```python
from build123d import *

# Parameters (mm, degrees)
SKETCH1_W           = 63.5
SKETCH1_H           = 38.1
BOSS_EXTRUDE1_DEPTH = 8.89
SKETCH2_R           = 2.4638
SKETCH2_R_2         = 1.5875
CUT_EXTRUDE1_DEPTH  = 7.366
SKETCH3_R           = 2.4638
SKETCH3_R_2         = 1.5875
CUT_EXTRUDE2_DEPTH  = 75.584798049


with BuildPart() as part:
    # Sketch1 → Boss-Extrude1 (new body)
    with BuildSketch(Plane(origin=(0, 0, 0), x_dir=(1, 0, 0), z_dir=(0, 1, 0))):
        with Locations((31.75, 19.05)):
            Rectangle(SKETCH1_W, SKETCH1_H)
    extrude(amount=BOSS_EXTRUDE1_DEPTH)

    # Sketch2 → Cut-Extrude1 (cut)
    # profile 1 of 6: a face of its own
    with BuildSketch(Plane(origin=(0, 8.89, 0), x_dir=(1, 0, 0), z_dir=(0, 1, 0))):
        Polygon((17.576011698, 25.4), (15.138005849, 29.62275), (10.261994151, 29.62275), (7.823988302, 25.4), (10.261994151, 21.17725), (15.138005849, 21.17725), align=None)
        with Locations(Location((12.7, 25.4, 0), (0, 0, 270))):
            Circle(SKETCH2_R, mode=Mode.SUBTRACT)
    # profile 2 of 6: a face of its own
    with BuildSketch(Plane(origin=(0, 8.89, 0), x_dir=(1, 0, 0), z_dir=(0, 1, 0))):
        Polygon((36.626011698, 25.4), (34.188005849, 29.62275), (29.311994151, 29.62275), (26.873988302, 25.4), (29.311994151, 21.17725), (34.188005849, 21.17725), align=None)
        with Locations(Location((31.75, 25.4, 0), (0, 0, 270))):
            Circle(SKETCH2_R, mode=Mode.SUBTRACT)
    # profile 3 of 6: a face of its own
    with BuildSketch(Plane(origin=(0, 8.89, 0), x_dir=(1, 0, 0), z_dir=(0, 1, 0))):
        Polygon((55.676011698, 25.4), (53.238005849, 29.62275), (48.361994151, 29.62275), (45.923988302, 25.4), (48.361994151, 21.17725), (53.238005849, 21.17725), align=None)
        with Locations(Location((50.8, 25.4, 0), (0, 0, 270))):
            Circle(SKETCH2_R, mode=Mode.SUBTRACT)
    # profile 4 of 6: a face of its own
    with BuildSketch(Plane(origin=(0, 8.89, 0), x_dir=(1, 0, 0), z_dir=(0, 1, 0))):
        Polygon((16.659468146, 12.7), (14.679734073, 16.129), (10.720265927, 16.129), (8.740531854, 12.7), (10.720265927, 9.271), (14.679734073, 9.271), align=None)
        with Locations(Location((12.7, 12.7, 0), (0, 0, 270))):
            Circle(SKETCH2_R_2, mode=Mode.SUBTRACT)
    # profile 5 of 6: a face of its own
    with BuildSketch(Plane(origin=(0, 8.89, 0), x_dir=(1, 0, 0), z_dir=(0, 1, 0))):
        Polygon((35.709468146, 12.7), (33.729734073, 16.129), (29.770265927, 16.129), (27.790531854, 12.7), (29.770265927, 9.271), (33.729734073, 9.271), align=None)
        with Locations(Location((31.75, 12.7, 0), (0, 0, 270))):
            Circle(SKETCH2_R_2, mode=Mode.SUBTRACT)
    # profile 6 of 6: a face of its own
    with BuildSketch(Plane(origin=(0, 8.89, 0), x_dir=(1, 0, 0), z_dir=(0, 1, 0))):
        Polygon((54.759468146, 12.7), (52.779734073, 16.129), (48.820265927, 16.129), (46.840531854, 12.7), (48.820265927, 9.271), (52.779734073, 9.271), align=None)
        with Locations(Location((50.8, 12.7, 0), (0, 0, 270))):
            Circle(SKETCH2_R_2, mode=Mode.SUBTRACT)
    extrude(amount=-CUT_EXTRUDE1_DEPTH, mode=Mode.SUBTRACT)

    # Sketch3 → Cut-Extrude2 (cut, through all)
    with BuildSketch(Plane(origin=(0, 8.89, 0), x_dir=(1, 0, 0), z_dir=(0, 1, 0))):
        with Locations(Location((12.7, 25.4, 0), (0, 0, 270))):
            Circle(SKETCH3_R)
        with Locations(Location((31.75, 25.4, 0), (0, 0, 270))):
            Circle(SKETCH3_R)
        with Locations(Location((50.8, 25.4, 0), (0, 0, 270))):
            Circle(SKETCH3_R)
        with Locations(Location((50.8, 12.7, 0), (0, 0, 270))):
            Circle(SKETCH3_R_2)
        with Locations(Location((31.75, 12.7, 0), (0, 0, 270))):
            Circle(SKETCH3_R_2)
        with Locations(Location((12.7, 12.7, 0), (0, 0, 270))):
            Circle(SKETCH3_R_2)
    extrude(amount=-CUT_EXTRUDE2_DEPTH, mode=Mode.SUBTRACT)


solid = part.part
```
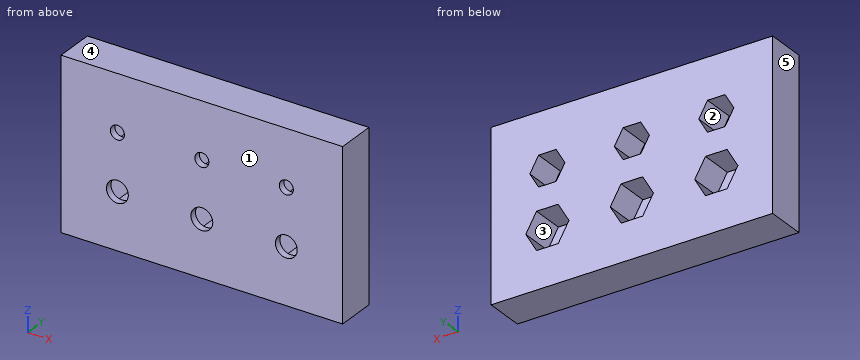
Work out the finished part from the listing and answer in its coordinate system (mm). Face numbers are marked on the shaded views. A direction names the side the tool comes from. Coordinates: 2 decimals unless noted, no trailing zeros. Loops run counter-clockwise (first coordinate to the right, second up) from the corner with the lowest first, then second, coordinate; pieces in that order, holes last. Notation, with made-up numbers: (44.25, 53) - (89.25, 53) arc R24 ccw to (89.25, 82) - close; hole circle Ø3 at (43.5, 8.25). An arc over 180 degrees is marked (long way). Use a Markdown table: item, result.
Item 1: For the marked faces 1 and 2, determine the directions among +Z, -Z, +X, -X, +Y, -Y from which every point of the face is accessible in a straight line to the end or side of a thin tool.
Evaluation:
| item | result |
|---|---|
| face 1 | +Z, -Z, +X, -X, -Y |
| face 2 | +Y |
Item 2: Find section B-B, the plane z = -24.5. Determine the outline of the cut face in (x, y).
Evaluation:
| item | result |
|---|---|
| outline | (0, 0) - (10.41, 0) - (10.41, 1.52) - (8.34, 1.52) - (8.34, 8.89) - (0, 8.89) - close; (14.99, 0) - (29.46, 0) - (29.46, 1.52) - (27.39, 1.52) - (27.39, 8.89) - (17.06, 8.89) - (17.06, 1.52) - (14.99, 1.52) - close; (34.04, 0) - (48.51, 0) - (48.51, 1.52) - (46.44, 1.52) - (46.44, 8.89) - (36.11, 8.89) - (36.11, 1.52) - (34.04, 1.52) - close; (53.09, 0) - (63.5, 0) - (63.5, 8.89) - (55.16, 8.89) - (55.16, 1.52) - (53.09, 1.52) - close |
Item 3: The mould has two halves that part along X. Classify the marked faces 3, 4 and 5: +X half, -X half, draft (parallel to the pull), parting line (faces both ways), or undercut.
Evaluation:
| item | result |
|---|---|
| face 3 | undercut |
| face 4 | draft |
| face 5 | -X half |
Item 4: Find section A-A, the plane x = 12.7. Determine the outline of the cut face in (y, z).
Evaluation:
| item | result |
|---|---|
| outline | (0, -38.1) - (8.89, -38.1) - (8.89, -29.62) - (1.52, -29.62) - (1.52, -27.86) - (0, -27.86) - close; (0, -22.94) - (1.52, -22.94) - (1.52, -21.18) - (8.89, -21.18) - (8.89, -16.13) - (1.52, -16.13) - (1.52, -14.29) - (0, -14.29) - close; (0, -11.11) - (1.52, -11.11) - (1.52, -9.27) - (8.89, -9.27) - (8.89, 0) - (0, 0) - close |
Item 5: Consider probe 1 along Z at (x, y) = (32, 6.25); probe 2 along X at (y, z) = (0.5, -12.7); probe 3 along X at (y, z) = (5.75, -24.5). Determine where each line is inside the solid, lowest interval first. Write a range as from..to.
Evaluation:
| item | result |
|---|---|
| probe 1 | z = -38.1..-29.62, -21.18..-16.13, -9.27..0 |
| probe 2 | x = 0..11.11, 14.29..30.16, 33.34..49.21, 52.39..63.5 |
| probe 3 | x = 0..8.34, 17.06..27.39, 36.11..46.44, 55.16..63.5 |
Item 6: Find section C-C, the plane z = -15. Determine the outline of the cut face in (x, y), and give its area (3 significant figures).
Evaluation:
| item | result |
|---|---|
| outline | (0, 0) - (63.5, 0) - (63.5, 8.89) - (53.43, 8.89) - (53.43, 1.52) - (48.17, 1.52) - (48.17, 8.89) - (34.38, 8.89) - (34.38, 1.52) - (29.12, 1.52) - (29.12, 8.89) - (15.33, 8.89) - (15.33, 1.52) - (10.07, 1.52) - (10.07, 8.89) - (0, 8.89) - close |
| area | 448 mm2 |
Item 7: Find section D-D, the plane y = 7. State how many separate pieces and enclosed holes the cut face has, and give its area (3 significant figures).
Evaluation:
| item | result |
|---|---|
| separate pieces | 1 |
| enclosed holes | 6 |
| area | 2,110 mm2 |
